from build123d import *

# Parameters (mm, degrees)
SKETCH1_W                       = 460
SKETCH1_H                       = 260
BASE_FLANGE1_DEPTH              = 10
BREAK_CORNER1_DEPTH             = 10
M10_CLEARANCE_HOLE1_D           = 12
M10_CLEARANCE_HOLE1_CSINK_D     = 12.05
M10_CLEARANCE_HOLE1_CSINK_ANGLE = 90
FILLET1_R                       = 3


# Read off the part's stored shape, not the designer's step: Break-Corner1
# Sheet-metal steps are written as plain solids
with BuildPart() as part:
    # Sketch1 → Base-Flange1 (new body)
    with BuildSketch(Plane(origin=(0, 0, 0), x_dir=(1, 0, 0), z_dir=(0, 1, 0))):
        Rectangle(SKETCH1_W, SKETCH1_H)
    extrude(amount=BASE_FLANGE1_DEPTH)

    # Break-Corner1 outline → Break-Corner1 (cut)
    with BuildSketch(Plane(origin=(0, 0, 0), x_dir=(1, 0, 0), z_dir=(0, 1, 0))):
        Polygon((230, -130), (230, -120), (220, -130), align=None)
        Polygon((220, 130), (230, 120), (230, 130), align=None)
    extrude(amount=BREAK_CORNER1_DEPTH, mode=Mode.SUBTRACT)

    # M10 Clearance Hole1 (through all)
    with Locations(Plane(origin=(0, 10, 0), x_dir=(1, 0, 0), z_dir=(0, 1, 0))):
        with Locations((-110, 78), (-10, 78), (90, 78), (-60, 26), (40, 26), (-60, -26), (40, -26), (-110, -78), (-10, -78), (90, -78)):
            CounterSinkHole(M10_CLEARANCE_HOLE1_D / 2, M10_CLEARANCE_HOLE1_CSINK_D / 2, counter_sink_angle=M10_CLEARANCE_HOLE1_CSINK_ANGLE)

    # Fillet1
    fillet1_edges = [part.edges().sort_by_distance(p)[0] for p in [
        (230, 0, 0),
        (230, 10, 0),
        (230, 5, 120),
        (225, 0, 125),
        (220, 5, 130),
        (225, 10, 125),
        (-5, 0, -130),
        (-5, 10, -130),
        (220, 5, -130),
        (225, 0, -125),
        (230, 5, -120),
        (225, 10, -125),
        (-5, 0, 130),
        (-230, 5, -130),
        (-230, 5, 130),
        (-5, 10, 130),
    ]]
    fillet(fillet1_edges, radius=FILLET1_R)


solid = part.part
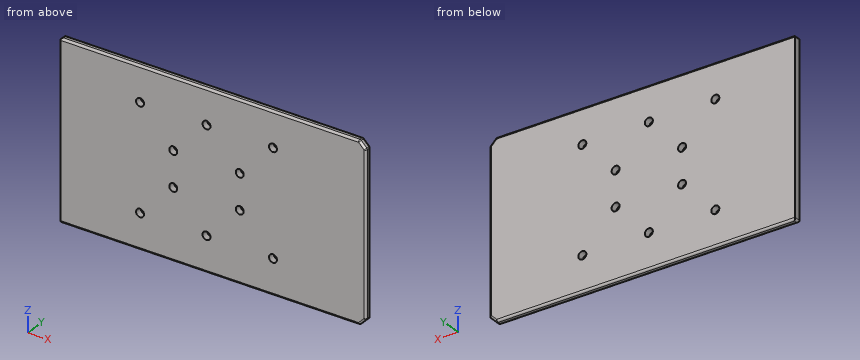
Could you check a few things on this model? Use its own coordinates, in mm. Coordinates: 2 decimals unless noted, no trailing zeros. Order: outer loops, then holes, each group sorted by start corner. A loop starts at its lowest first (then second) coordinate and runs counter-clockwise, first axis right, second up. Notation, with made-up numbers: (-16.75, -16) - (18.25, -16) arc R22 ccw to (18.25, -7) - close; hole circle Ø6 at (9, -1.75). An arc over 180 degrees is marked (long way). Answer in a Markdown table with one row per item. Add a question column.
(1) Will this pin go through, and if not, where does the flat tip stop? pin 1 (7 mm diameter, centred on x = 90, z = 78, fed in from -Y).
(2) If we section it at C-C, the plane z = 78: Please give me the cut outline in (x, y) (3 decimals).
(3) I need wall thicknesses on L1, parallel to Z at x = -60, y = 3.75; L2, parallel to X at y = 6.5, z = 78; L3, parallel to Z at x = -110, y = 3. Which ranges of each line are inside material? Lowest first, please.
(4) If we section it at B-B, the plane x = -110: Please give me the cut outline in (y, z) (3 decimals).
(5) If we section it at A-A, the plane z = 26: Please give me the cut outline in (x, y) (3 decimals), then the cut area to 3 significant figures.
Results are:
| question | item | result |
|---|---|---|
| 1 | pin 1 | passes through |
| 2 | outline | (-230, 0) - (-116, 0) - (-116, 9.975) - (-116.025, 10) - (-230, 10) - close; (-104, 0) - (-16, 0) - (-16, 9.975) - (-16.025, 10) - (-103.975, 10) - (-104, 9.975) - close; (-4, 0) - (84, 0) - (84, 9.975) - (83.975, 10) - (-3.975, 10) - (-4, 9.975) - close; (96, 0) - (227, 0) arc R3 ccw to (230, 3) - (230, 7) arc R3 ccw to (227, 10) - (96.025, 10) - (96, 9.975) - close |
| 3 | L1 | z = -130 to -32, -20 to 20, 32 to 130 |
| 3 | L2 | x = -230 to -116, -104 to -16, -4 to 84, 96 to 230 |
| 3 | L3 | z = -130 to -84, -72 to 72, 84 to 130 |
| 4 | outline | (0, -127) arc R3 ccw to (3, -130) - (7, -130) arc R3 ccw to (10, -127) - (10, -84.025) - (9.975, -84) - (0, -84) - close; (0, -72) - (9.975, -72) - (10, -71.975) - (10, 71.975) - (9.975, 72) - (0, 72) - close; (0, 84) - (9.975, 84) - (10, 84.025) - (10, 127) arc R3 ccw to (7, 130) - (3, 130) arc R3 ccw to (0, 127) - close |
| 5 | outline | (-230, 0) - (-66, 0) - (-66, 9.975) - (-66.025, 10) - (-230, 10) - close; (-54, 0) - (34, 0) - (34, 9.975) - (33.975, 10) - (-53.975, 10) - (-54, 9.975) - close; (46, 0) - (227, 0) arc R3 ccw to (230, 3) - (230, 7) arc R3 ccw to (227, 10) - (46.025, 10) - (46, 9.975) - close |
| 5 | area | 4,360 mm2 |
